Design review of the part built by this model. Coordinates are the model's own, in mm. A direction names the side the tool comes from. Coordinates: 2 decimals unless noted, no trailing zeros. Loops run counter-clockwise (first coordinate to the right, second up) from the corner with the lowest first, then second, coordinate; pieces in that order, holes last. Notation, with made-up numbers: (-10, -28.75) -> (28, -28.75) arc R22 cw to (28, 3.25) -> close; hole circle Ø8 at (-5.75, 34). An arc over 180 degrees is marked (long way). Use CSV: the item, a comma, the result in double quotes.
```python
from build123d import *

# Parameters (mm, degrees)
F0_W     = 179
F0_H     = 94
F0_W_2   = 82
F0_H_2   = 49.999998
F1_DEPTH = 35
F2_DEPTH = 15


with BuildPart() as f1:
    # F0 (on Top) → F1 (new body)
    with BuildSketch(Plane.XY):
        Rectangle(F0_W, F0_H)
        Polygon((-79.489959, -29.920486), (-78.995136, -30.08246), (-78.53955, -30.334507), (-78.1386, -31.012478), (-74.467219, -37.220443), (-74.45244, -37.585563), (-74.445794, -37.74979), (-74.527791, -38.273187), (-74.710072, -38.77062), (-74.985671, -39.223072), (-75.344048, -39.613243), (-75.7715, -39.926215), (-76.251686, -40.15002), (-76.766246, -40.276102), (-77.295502, -40.29964), (-77.819223, -40.219734), (-78.31738, -40.039439), (-78.770929, -39.765649), (-82.84326, -32.879713), (-82.84465, -32.359057), (-82.748207, -31.847408), (-82.557362, -31.362987), (-82.278913, -30.923042), (-81.922774, -30.543238), (-81.501627, -30.237101), (-81.030467, -30.015529), (-80.526071, -29.886415), (-80.006401, -29.854352), align=None, mode=Mode.SUBTRACT)
        Polygon((82.808956, -32.243232), (82.818469, -32.763804), (78.891239, -39.733514), (78.443523, -40.016743), (77.949251, -40.207431), (77.427319, -40.298287), (76.897685, -40.285837), (76.380599, -40.17056), (75.895831, -39.956859), (75.461917, -39.652909), (75.095447, -39.270329), (74.810434, -38.823747), (74.617775, -38.33024), (74.524835, -37.808676), (74.530136, -37.537048), (74.53517, -37.278996), (78.125485, -30.907213), (78.4624, -30.309285), (78.912607, -30.047753), (79.403929, -29.875452), (79.918872, -29.798517), (80.439101, -29.819689), (80.946089, -29.938213), (81.421786, -30.149868), (81.849253, -30.447118), (82.213267, -30.81938), (82.500869, -31.253398), (82.701817, -31.733715), align=None, mode=Mode.SUBTRACT)
        with Locations((-11.5, 0)):
            Rectangle(F0_W_2, F0_H_2, mode=Mode.SUBTRACT)
        Polygon((-74.745494, 38.78665), (-74.544546, 38.306332), (-74.437408, 37.796815), (-74.432649, 37.536394), (-74.427894, 37.276243), (-78.019246, 30.902619), (-78.355124, 30.306533), (-78.80284, 30.023304), (-79.297113, 29.832617), (-79.819044, 29.741761), (-80.348679, 29.75421), (-80.865765, 29.869488), (-81.350532, 30.083188), (-81.784446, 30.387139), (-82.150917, 30.769718), (-82.435929, 31.2163), (-82.628588, 31.709807), (-82.721528, 32.231372), (-82.711193, 32.761052), (-78.783964, 39.730762), (-78.333757, 39.992295), (-77.842433, 40.164595), (-77.32749, 40.24153), (-76.807263, 40.220358), (-76.300273, 40.101835), (-75.824577, 39.890179), (-75.397111, 39.592929), (-75.033095, 39.220667), align=None, mode=Mode.SUBTRACT)
        Polygon((78.240855, 39.942996), (78.69644, 39.690949), (82.768772, 32.805012), (82.790197, 32.275666), (82.708201, 31.752269), (82.525919, 31.254834), (82.250321, 30.802382), (81.891943, 30.412212), (81.464491, 30.099241), (80.984305, 29.875435), (80.469745, 29.749353), (79.940489, 29.725815), (79.416768, 29.805721), (78.918611, 29.986015), (78.465062, 30.259805), (78.062882, 30.939855), (74.39273, 37.145741), (74.391731, 37.519846), (74.391341, 37.666399), (74.487784, 38.178047), (74.678629, 38.662468), (74.957078, 39.102413), (75.313217, 39.482216), (75.734364, 39.788353), (76.205524, 40.009925), (76.70992, 40.139041), (77.22959, 40.171102), (77.746032, 40.104968), align=None, mode=Mode.SUBTRACT)
    extrude(amount=F1_DEPTH)

    # F0 (on Top) → F2 (join)
    with BuildSketch(Plane.XY):
        with Locations((-11.5, 0)):
            Rectangle(F0_W_2, F0_H_2)
    extrude(amount=F2_DEPTH)


solid = f1.part
```
Item 1: Clearance check with flat-ended pins moving along their axes: pin 1 (4 mm diameter, centred on x = -25, y = -17.5, fed in from -Z); pin 2 (25 mm diameter, centred on x = -31.5, y = 9.5, fed in from +Z). State where each tip first meets the part, or that it passes through.
Checked values:
pin 1,"z = 0"
pin 2,"z = 15"
Item 2: Add section A-A (y = -9). Give the boundary of the cut face in (x, z).
Checked values:
outline,"(-89.5, 0) -> (89.5, 0) -> (89.5, 35) -> (29.5, 35) -> (29.5, 15) -> (-52.5, 15) -> (-52.5, 35) -> (-89.5, 35) -> close"
Item 3: To check wall thickness, follow line 1 along X through (y, z) = (-20, 19.5); line 2 along Y through (x, z) = (9, 32); line 3 along X through (y, z) = (-39, 21.5). State the ranges of each line that lie inside material, in increasing order.
Checked values:
line 1,"-89.5 to -52.5, 29.5 to 89.5"
line 2,"-47 to -25, 25 to 47"
line 3,"-89.5 to -79.22, -74.85 to 74.92, 79.3 to 89.5"
Item 4: Draft analysis for pull direction Y (two halves, no side actions). For faces 4 (the face through (-80.775, 36.197, 17.255)), 5 (the face through (-1, 47, 17)), 6 (the face through (-1, -47, 17)), state which applies: pulls with the +Y half, pulls with the -Y half, needs draft (parallel to the pull), parting line crosses it, or undercut.
Checked values:
face 4,"undercut"
face 5,"pulls with the +Y half"
face 6,"pulls with the -Y half"
Item 5: Add section C-C (z = 30). State how many separate pieces and enclosed holes the cut face has, then the cut area to 3 significant figures.
Checked values:
separate pieces,"1"
enclosed holes,"5"
area,"12,500 mm^2"
Item 6: Add section B-B (x = 21.5). Give the boundary of the cut face in (y, z), then the cut area to 3 significant figures.
Checked values:
outline,"(-47, 0) -> (47, 0) -> (47, 35) -> (25, 35) -> (25, 15) -> (-25, 15) -> (-25, 35) -> (-47, 35) -> close"
area,"2,290 mm^2"
Item 7: Machinability: for faces 1 (the face through (29.5, 0, 25)), 2 (the face through (89.5, -1, 17)), 3 (the face through (80.7, 36.3, 17.3)), which of the approach directions +Z, -Z, +X, -X, +Y, -Y give a long, thin tool a straight path to every point of the face, cutting with its end or side? Answer none if there is none.
Checked values:
face 1,"+Z"
face 2,"+Z, -Z, +X, +Y, -Y"
face 3,"+Z, -Z"
